Autodesk Inventor part; units mm, degrees
ref_plane "YZ Plane" through (0, 0, 0) normal (1, 0, 0) x (0, 1, 0)
ref_plane "XZ Plane" through (0, 0, 0) normal (0, 1, 0) x (-1, 0, 0)
ref_plane "XY Plane" through (0, 0, 0) normal (0, 0, 1) x (1, 0, 0)
sketch "Sketch1" plane through (0, 0, 0) normal (0, 1, 0) x (-1, 0, 0)
  arc A0 (-19.05, 0) -> (19.05, 0) centre (0, 0) ccw
  line L0 (19.05, 0) -> (-19.05, 0)
revolve "Revolution1" add sketch "Sketch1" angle 180 about axis through (-19.05, 0, 0) along (1, 0, 0)
sketch "Sketch2" plane through (0, 0, 0) normal (0, -1, 0) x (1, 0, 0)
  circle A0 centre (0, 0) radius 19.05
extrude "Extrusion1" add sketch "Sketch2" along normal blind 8.89
sketch "Sketch3" plane through (0, 0, 0) normal (1, 0, 0) x (0, 1, 0)
  line L0 (-8.89, 19.05) -> (-8.89, -19.05)
  line L1 (-8.89, 0) -> (-72.39, 0)
  arc A0 (-72.39, 37.2434) -> (-8.89, 19.05) centre (-8.89, 138.9628) ccw
  arc A1 (-72.39, 34.643) -> (-8.89, 16.8363) centre (-8.89, 138.9628) ccw
  line L2 (-8.89, 16.8363) -> (0, 16.8363)
  line L3 (-72.39, 37.2434) -> (-72.39, 34.643)
  line L4 (-8.89, 16.8363) -> (-8.89, 19.05)
  point P0 (0, 0)
  point P1 (-8.89, 16.8363)
  dimension "d4" = 63.5
revolve "Revolution2" add sketch "Sketch3" angle 360 about axis through (0, -8.89, 0) along (0, -1, 0)
properties part number "cock1"
Can you work these out from the model? Positions are in its coordinate system, mm. Round coordinates to 2 decimals unless told otherwise and drop trailing zeros. Order: outer loops, then holes, each group sorted by start corner. A loop starts at its lowest first (then second) coordinate and runs counter-clockwise, first axis right, second up.
(1) If we section it at D-D (y = 9): Please give me the cut outline in (x, z).
Results are:
outline: circle Ø33.58 at (0, 0)
(2) I'm going to push flat-ended pins straight in: pin 1 (6 mm diameter, centred on y = -11.5, z = -13.5, fed in from +X); pin 2 (6 mm diameter, centred on x = -8, z = -19, fed in from +Y); pin 3 (1.5 mm diameter, centred on y = -47.5, z = -24, fed in from -X); pin 4 (12 mm diameter, centred on y = -2.5, z = -26.5, fed in from -X). Where does each tip first touch, or does it pass through?
Results are:
pin 1: stops at x = 15.93
pin 2: stops at y = 7.25
pin 3: stops at x = -10.43
pin 4: passes through
(3) If we section it at C-C (y = -60): Please give me the cut outline in (x, z), plus the area to 3 significant figures.
Results are:
outline: circle Ø60.98 at (0, 0); hole circle Ø56.09 at (0, 0)
area: 449 mm2
(4) If we section it at A-A (z = 0): Please give me the cut outline in (x, y), plus the area to 3 significant figures.
Results are:
outline: (-37.24, -72.39) - (-34.64, -72.39) arc R122.13 ccw to (-16.84, -8.89) - (16.84, -8.89) arc R122.13 ccw to (34.64, -72.39) - (37.24, -72.39) arc R119.91 cw to (19.05, -8.89) - (19.05, 0) arc R19.05 ccw to (-19.05, 0) - (-19.05, -8.89) arc R119.91 cw to start
area: 1,200 mm2
(5) We'd pull the mould along Z, two halves only. Please class faces 1 (the face through (25, -72.39, 25)), 2 (the face through (0, -8.89, 0)), 3 (the face through (-15.12, -4.38, 11.59)): +Z half, -Z half, draft (parallel to the pull), parting line (faces both ways), or undercut.
Results are:
face 1: draft
face 2: undercut
face 3: parting line
(6) If I drill on L1, parallel to X at y = -36, z = 16; L2, parallel to Z at x = 20.5, y = -52.5; L3, parallel to Z at x = -28, y = -67.5, over which ranges is the centre line in solid material (lowest first)?
Results are:
L1: x = -15.32 to -11.8, 11.8 to 15.32
L2: z = -17.97 to -14.11, 14.11 to 17.97
L3: z = -19.9 to -15.12, 15.12 to 19.9
(7) If we section it at B-B (x = 0): Please give me the cut outline in (y, z), plus the area to 3 significant figures.
Results are:
outline: (-72.39, -37.24) arc R119.91 cw to (-8.89, -19.05) - (0, -19.05) arc R19.05 ccw to (0, 19.05) - (-8.89, 19.05) arc R119.91 cw to (-72.39, 37.24) - (-72.39, 34.64) arc R122.13 ccw to (-8.89, 16.84) - (-8.89, -16.84) arc R122.13 ccw to (-72.39, -34.64) - close
area: 1,200 mm2
